Geometry: see drawing. Coordinates: mm, zero at the bounding-box minimum. A direction names the side the tool comes from. Round coordinates to 2 decimals unless told otherwise and drop trailing zeros. Loops run counter-clockwise (first coordinate to the right, second up) from the corner with the lowest first, then second, coordinate; pieces in that order, holes last.
(1) Access query for the marked faces 1 and 2. Directions: +Z, -Z, +X, -X, +Y, -Y. A direction counts if a zero-diameter tool reaches every point of the face in a straight line with its end or side. Return the directions, or none.
(2) Line query: line 1 (Z direction, x = 10, y = 7.25); line 2 (Y direction, x = 18, z = 12); line 3 (Z direction, x = 7, y = 9). Output: solid intervals per line, ascending.
(3) First-contact query: pin 1 Ø1 at (x, y) = (13.5, 10.5) entering from +Z; pin 2 Ø5 at (y, z) = (6.5, 7) entering from -X; pin 3 Ø2 at (y, z) = (11, 4.5) entering from +X; pin 4 Ø6.5 at (x, z) = (10, 10) entering from -Y. Flat tips, straight axial feed; report the tip coordinate or a pass-through.
(4) Cut plane A-A, the plane z = 10. Output: boundary loops of the cut face in (x, y), and give its area (3 significant figures).
(5) Cut plane D-D, the plane x = 3.75. Output: boundary loops of the cut face in (y, z), and give its area (3 significant figures).
(6) Cut plane C-C, the plane y = 4.25. Output: boundary loops of the cut face in (x, z), and give its area (3 significant figures).
(7) Cut plane B-B, the plane x = 10. Output: boundary loops of the cut face in (y, z).
(8) Draft query along X for the marked faces 3, 4 and 5. Return one class per face: released by +X, released by -X, zero draft, split by the parting line, or undercut.
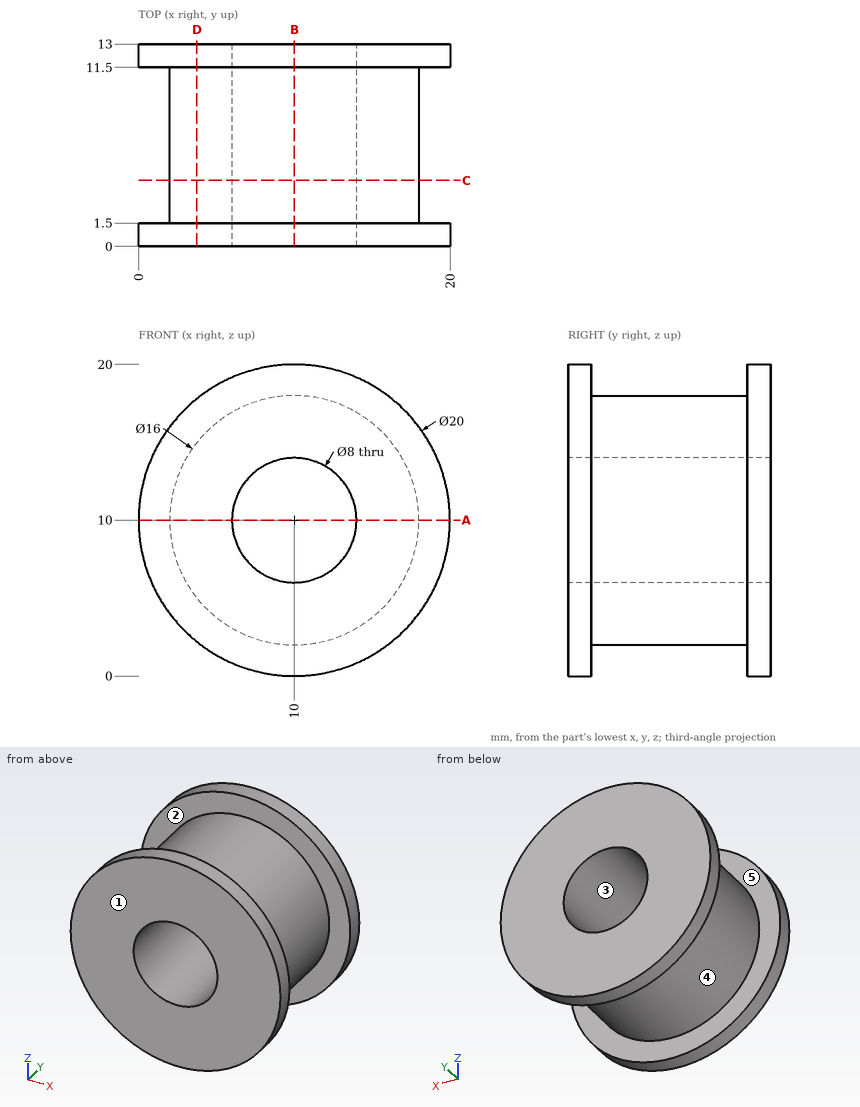
Reported:
1. face 1: +Z, -Z, +X, -X, -Y
1. face 2: none
2. line 1: z = 2 to 6, 14 to 18
2. line 2: y = 0 to 1.5, 11.5 to 13
2. line 3: z = 2.58 to 7.35, 12.65 to 17.42
3. pin 1: stops at z = 17.42
3. pin 2: stops at x = 2.02
3. pin 3: stops at x = 18.86
3. pin 4: passes through
4. outline: (0, 0) - (6, 0) - (6, 13) - (0, 13) - (0, 11.5) - (2, 11.5) - (2, 1.5) - (0, 1.5) - close; (14, 0) - (20, 0) - (20, 1.5) - (18, 1.5) - (18, 11.5) - (20, 11.5) - (20, 13) - (14, 13) - close
4. area: 116 mm2
5. outline: (0, 2.19) - (1.5, 2.19) - (1.5, 5.01) - (11.5, 5.01) - (11.5, 2.19) - (13, 2.19) - (13, 17.81) - (11.5, 17.81) - (11.5, 14.99) - (1.5, 14.99) - (1.5, 17.81) - (0, 17.81) - close
5. area: 147 mm2
6. outline: circle Ø16 at (10, 10); hole circle Ø8 at (10, 10)
6. area: 151 mm2
7. outline: (0, 0) - (1.5, 0) - (1.5, 2) - (11.5, 2) - (11.5, 0) - (13, 0) - (13, 6) - (0, 6) - close; (0, 14) - (13, 14) - (13, 20) - (11.5, 20) - (11.5, 18) - (1.5, 18) - (1.5, 20) - (0, 20) - close
8. face 3: undercut
8. face 4: split by the parting line
8. face 5: zero draft
